Can you work these out from the model? Positions are in its coordinate system, mm. A direction names the side the tool comes from. Give positions to 0.01 mm unless a question says otherwise; leave off trailing zeros. Order: outer loops, then holes, each group sorted by start corner. A loop starts at its lowest first (then second) coordinate and runs counter-clockwise, first axis right, second up. Notation, with made-up numbers: (47.25, 59) - (65.25, 59) arc R38 ccw to (65.25, 97) - close; hole circle Ø4 at (-12, -31). An arc over 180 degrees is marked (long way). Answer as CSV lines item,"result".
```python
from build123d import *

# Parameters (mm, degrees)
F0_W     = 160
F0_H     = 75
F0_R     = 17.5
F1_DEPTH = 15
F2_R     = 2.5
F2_R_2   = 19.05
F3_DEPTH = 25
F4_R     = 4
F5_DEPTH = 6
F6_W     = 60
F6_H     = 5
F7_DEPTH = 79.7


# Not quite as in the source:
# - a feature names something its author has since deleted; it is built from what else it names


with BuildPart() as f1:
    # F0 (on Top) → F1 (new body)
    with BuildSketch(Plane.XY):
        Rectangle(F0_W, F0_H)
        Circle(F0_R, mode=Mode.SUBTRACT)
    extrude(amount=F1_DEPTH)

    # F2 (on face) → F3 (cut)
    with BuildSketch(Plane.XY.offset(15)):
        with Locations((-73.55, 23.55)):
            Circle(F2_R)
        with Locations((-26.45, 23.55)):
            Circle(F2_R)
        with Locations((-26.45, -23.55)):
            Circle(F2_R)
        with Locations((-73.55, -23.55)):
            Circle(F2_R)
        with Locations((-50, 0)):
            Circle(F2_R_2)
    extrude(amount=-F3_DEPTH, mode=Mode.SUBTRACT)

    # F4 (on face) → F5 (cut)
    with BuildSketch(Plane(origin=(0, 0, 0), x_dir=(1, 0, 0), z_dir=(0, 0, -1))):
        with Locations((-73.55, 23.55)):
            Circle(F4_R)
        with Locations((-26.45, 23.55)):
            Circle(F4_R)
        with Locations((-26.45, -23.55)):
            Circle(F4_R)
        with Locations((-73.55, -23.55)):
            Circle(F4_R)
    extrude(amount=-F5_DEPTH, mode=Mode.SUBTRACT)

    # F6 (on face) → F7 (cut)
    with BuildSketch(Plane.XZ.offset(37.5)):
        with Locations((-50, 2.5)):
            Rectangle(F6_W, F6_H)
    extrude(amount=-F7_DEPTH, mode=Mode.SUBTRACT)


solid = f1.part
```
1) I want a section at B-B on x = 0. Write out the boundary of the cut face in (y, z), plus the area to 3 significant figures.
Answer block:
outline,"(-37.5, 0) - (-17.5, 0) - (-17.5, 15) - (-37.5, 15) - close; (17.5, 0) - (37.5, 0) - (37.5, 15) - (17.5, 15) - close"
area,"600 mm2"
2) I want a section at A-A on y = -23.55. Write out the boundary of the cut face in (x, z), plus the area to 3 significant figures.
Answer block:
outline,"(-80, 5) - (-77.55, 5) - (-77.55, 6) - (-76.05, 6) - (-76.05, 15) - (-80, 15) - close; (-71.05, 6) - (-69.55, 6) - (-69.55, 5) - (-30.45, 5) - (-30.45, 6) - (-28.95, 6) - (-28.95, 15) - (-71.05, 15) - close; (-23.95, 6) - (-22.45, 6) - (-22.45, 5) - (-20, 5) - (-20, 0) - (80, 0) - (80, 15) - (-23.95, 15) - close"
area,"1,990 mm2"
3) I'm going to push flat-ended pins straight in: P1, Ø2.5, axis at x = -72, y = -24, coming from the -Z side; P2, Ø6.5, axis at x = -74, y = 22, coming from the -Z side; P3, Ø1.5, axis at y = 0, z = 2, coming from the -X side. Where does each tip first touch, or does it pass through?
Answer block:
P1,"z = 6"
P2,"z = 5"
P3,"x = -20"
4) If we mould it in two halves opening along X, with no side actions, what happens to faces 4 (the flat face through (-73.6, 26.2, 6)), 5 (the flat face through (29, 1, 0)), 6 (the flat face through (80, -1, 7))? For each: +X half, -X half, draft (parallel to the pull), parting line (faces both ways), or undercut.
Answer block:
face 4,"undercut"
face 5,"draft"
face 6,"+X half"
5) I want a section at C-C on z = 3.5. Write out the boundary of the cut face in (x, y), plus the area to 3 significant figures.
Answer block:
outline,"(-20, -37.5) - (80, -37.5) - (80, 37.5) - (-20, 37.5) - close; hole circle Ø35 at (0, 0)"
area,"6,540 mm2"
6) I want a section at D-D on x = -26.45. Write out the boundary of the cut face in (y, z), plus the area to 3 significant figures.
Answer block:
outline,"(-37.5, 5) - (-27.55, 5) - (-27.55, 6) - (-26.05, 6) - (-26.05, 15) - (-37.5, 15) - close; (-21.05, 6) - (-19.55, 6) - (-19.55, 5) - (19.55, 5) - (19.55, 6) - (21.05, 6) - (21.05, 15) - (-21.05, 15) - close; (26.05, 6) - (27.55, 6) - (27.55, 5) - (37.5, 5) - (37.5, 15) - (26.05, 15) - close"
area,"644 mm2"
7) I need wall thicknesses on line 1 along X through (y, z) = (23.55, 5.65); line 2 along Y through (x, z) = (-26.45, 9.5); line 3 along Y through (x, z) = (-50, 10.5). Which ranges of each line are inside material? Lowest first, please. Write a range as [from, to].
Answer block:
line 1,"[-80, -77.55], [-69.55, -30.45], [-22.45, 80]"
line 2,"[-37.5, -26.05], [-21.05, 21.05], [26.05, 37.5]"
line 3,"[-37.5, -19.05], [19.05, 37.5]"
8) Which directions (+Z, -Z, +X, -X, +Y, -Y) give clear straight access to the entire face, cutting with the end or side of a thin tool? Please do faces 1 (the flat face through (-20, -1, 2)), 2 (the cylindrical face through (-24.604, -20.001, 5.493)), 3 (the cylindrical face through (-13.887, -10.648, 7.395)).
Answer block:
face 1,"-Z, -X, +Y, -Y"
face 2,"-Z"
face 3,"+Z, -Z"
